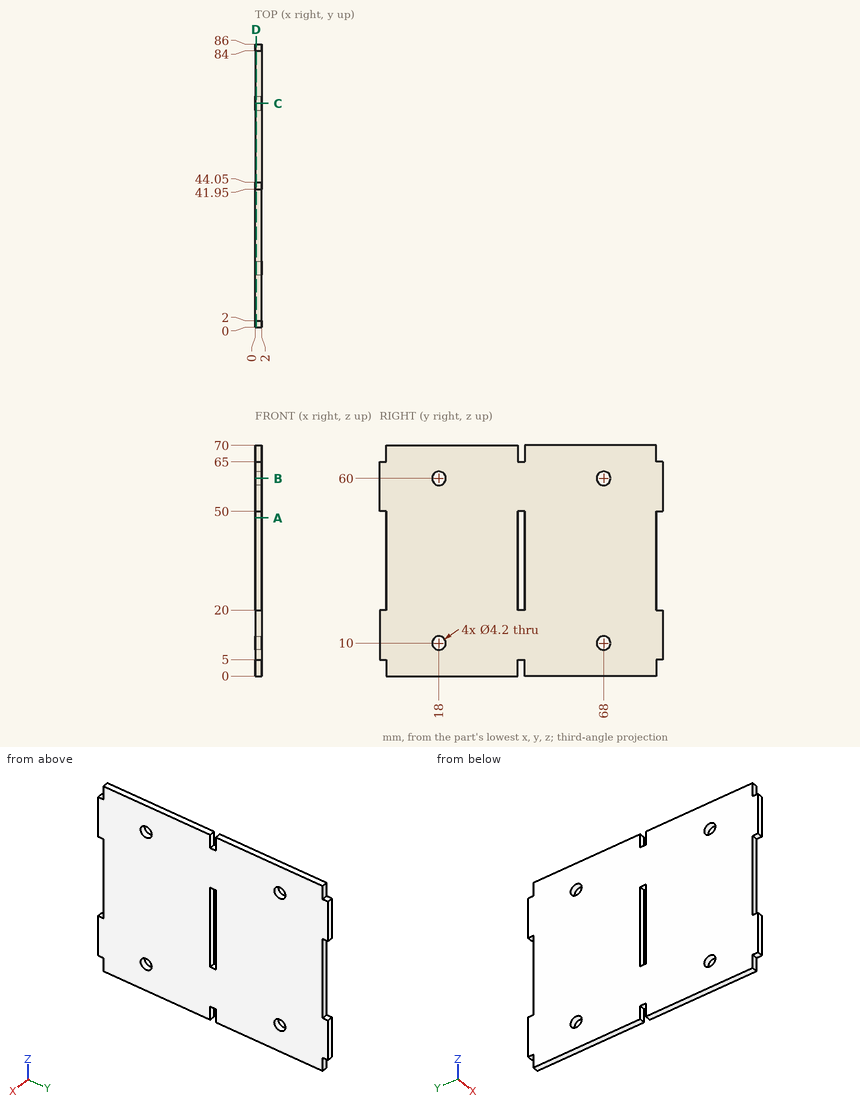
Could you check a few things on this drawing? It's one solid part, dimensions in mm from its lowest x, y, z. Give positions to 0.01 mm unless a question says otherwise; leave off trailing zeros. Order: outer loops, then holes, each group sorted by start corner. A loop starts at its lowest first (then second) coordinate and runs counter-clockwise, first axis right, second up.
1. I need wall thicknesses on L1, parallel to Y at x = 0.95, z = 60; L2, parallel to Y at x = 0.25, z = 30; L3, parallel to Y at x = 1.05, z = 59.5. Which ranges of each line are inside material? Lowest first, please.
Answers below:
L1: y = 0 to 15.9, 20.1 to 65.9, 70.1 to 86
L2: y = 2 to 41.95, 44.05 to 84
L3: y = 0 to 15.96, 20.04 to 65.96, 70.04 to 86
2. Suppose I cut it at A-A (z = 48). Write out the boundary of the cut face in (x, y).
Answers below:
outline: (0, 2) - (2, 2) - (2, 41.95) - (0, 41.95) - close; (0, 44.05) - (2, 44.05) - (2, 84) - (0, 84) - close
3. For pin 1 (0.6 mm diameter, centred on x = 1, y = 43, fed in from -Z); pin 2 (1 mm diameter, centred on x = 1, z = 67, fed in from -Y); pin 3 (0.6 mm diameter, centred on x = 0.5, z = 28.5, fed in from +Y), each with a flat end and sliding along its axis, tell me the tip position at first contact or that it passes through.
Answers below:
pin 1: stops at z = 5
pin 2: stops at y = 2
pin 3: stops at y = 84
4. Suppose I cut it at C-C (y = 68). Write out the boundary of the cut face in (x, z).
Answers below:
outline: (0, 0) - (2, 0) - (2, 7.9) - (0, 7.9) - close; (0, 12.1) - (2, 12.1) - (2, 57.9) - (0, 57.9) - close; (0, 62.1) - (2, 62.1) - (2, 70) - (0, 70) - close
5. Suppose I cut it at B-B (z = 60). Write out the boundary of the cut face in (x, y), plus the area to 3 significant figures.
Answers below:
outline: (0, 0) - (2, 0) - (2, 15.9) - (0, 15.9) - close; (0, 20.1) - (2, 20.1) - (2, 65.9) - (0, 65.9) - close; (0, 70.1) - (2, 70.1) - (2, 86) - (0, 86) - close
area: 155 mm2
6. Suppose I cut it at D-D (x = 0.35). State how many separate pieces and enclosed holes the cut face has, plus the area to 3 significant figures.
Answers below:
separate pieces: 1
enclosed holes: 5
area: 5,720 mm2
